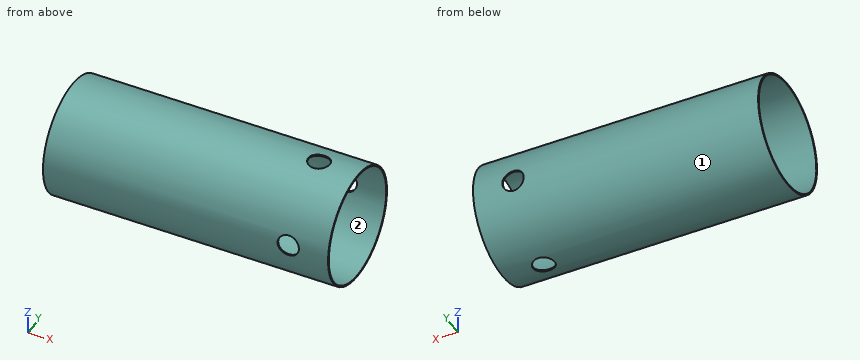
```python
from build123d import *

# Parameters (mm, degrees)
SKETCH014_R             = 8
PAD006_DEPTH            = 40
SKETCH015_R             = 1.5
POCKET008_DEPTH         = 11
POLARPATTERN002_COUNT   = 4
SKETCH016_R             = 7.8
POCKET009_DEPTH         = 40.001
BODY004_PLACEMENT_ANGLE = 87


with BuildPart() as part:
    # Sketch014 → Pad006 (new body)
    with BuildSketch(Plane.YZ.offset(10)):
        Circle(SKETCH014_R)
    extrude(amount=-PAD006_DEPTH)

    # Sketch015 → Pocket008 (cut)
    with BuildSketch(Plane.XY):
        with Locations((4.4, 0)):
            Circle(SKETCH015_R)
    pocket008 = extrude(amount=POCKET008_DEPTH, mode=Mode.SUBTRACT)

    # PolarPattern002: Pocket008 ×4 about axis
    polarpattern002_axis = Axis((0, 0, 0), (1, 0, 0))
    for i in range(1, POLARPATTERN002_COUNT):
        add(pocket008.rotate(polarpattern002_axis, i * 360 / POLARPATTERN002_COUNT), mode=Mode.SUBTRACT)

    # Sketch016 (on Face3 of Pad006) → Pocket009 (cut, through all)
    with BuildSketch(Plane(origin=(-30, 0, 0), x_dir=(0, 1, 0), z_dir=(-1, 0, 0))):
        Circle(SKETCH016_R)
    extrude(amount=-POCKET009_DEPTH, mode=Mode.SUBTRACT)


with BuildPart() as part_1:
    # Body004 placement: moved
    add(part.part.moved(Location((2, 0, 0))).rotate(Axis((2, 0, 0), (1, 0, 0)), BODY004_PLACEMENT_ANGLE))


solid = part_1.part
```
Check sheet for the modelled part. Datum: model origin and axes. Units: mm. Face numbers are marked on the shaded views. Round coordinates to 2 decimals unless told otherwise and drop trailing zeros. Loops run counter-clockwise (first coordinate to the right, second up) from the corner with the lowest first, then second, coordinate; pieces in that order, holes last. Notation, with made-up numbers: M 87,-23 L 101,-23 A27 ccw 101,0 Z; hole C -27.5,-14.75 d10. An arc over 180 degrees is marked long. Answer as a JSON object with one key per item and string values.
1. Scan lines: line 1 (Y direction, x = 1.5, z = 0); line 2 (Z direction, x = -4, y = -3). Record each from-to range of solid material in increasing order.
Reply:
{"line 1": "y = -8 to -7.8, 7.8 to 8", "line 2": "z = -7.42 to -7.2, 7.2 to 7.42"}
2. Section check B-B (z = -7). Record the boundary of the cut face in (x, y).
Reply:
{"outline": "M -28,-3.87 L 12,-3.87 L 12,-3.44 L -28,-3.44 Z; M -28,3.44 L 12,3.44 L 12,3.87 L -28,3.87 Z"}
3. Gauge pin test, flat ends, axial feed: P1, Ø2, axis at x = -10.5, z = 1.5, coming from the -Y side; P2, Ø1.5, axis at x = -16.5, z = -2, coming from the +Y side; P3, Ø2, axis at x = -9, z = 3.5, coming from the +Y side; P4, Ø1.5, axis at x = -4, y = -0.5, coming from the +Z side. Record the tip position at first contact, or that the pin passes through.
Reply:
{"P1": "stops at y = -7.98", "P2": "stops at y = 7.9", "P3": "stops at y = 7.6", "P4": "stops at z = 8"}
4. Section check A-A (y = -5). Record the boundary of the cut face in (x, z) (3 decimals).
Reply:
{"outline": "M -28,-6.245 L 12,-6.245 L 12,-5.987 L -28,-5.987 Z; M -28,5.987 L 12,5.987 L 12,6.245 L -28,6.245 Z"}
5. Section check C-C (x = 7). Record the boundary of the cut face in (y, z).
Reply:
{"outline": "M -7.94,-0.96 A8 ccw -1.79,-7.8 L -1.77,-7.6 A7.8 cw -7.74,-0.97 Z; M -7.8,1.79 L -7.6,1.77 A7.8 cw -0.97,7.74 L -0.96,7.94 A8 ccw Z; M 0.96,-7.94 A8 ccw 7.8,-1.79 L 7.6,-1.77 A7.8 cw 0.97,-7.74 Z; M 1.77,7.6 A7.8 cw 7.74,0.97 L 7.94,0.96 A8 ccw 1.79,7.8 Z"}
6. Section check D-D (z = 0). State how many separate pieces and enclosed holes the cut face has, plus the area to 3 significant figures.
Reply:
{"separate pieces": "4", "enclosed holes": "0", "area": "14.8 mm²"}
7. Mould release check, pull along Y, two halves, no side actions. Record for the marked faces 1 and 2: pulls with the +Y half, pulls with the -Y half, needs draft (parallel to the pull), parting line crosses it, or undercut.
Reply:
{"face 1": "parting line crosses it", "face 2": "undercut"}
